from build123d import *

# Parameters (mm, degrees)
SKETCH1_R           = 1.625
BOSS_EXTRUDE1_DEPTH = 6.35


with BuildPart() as part:
    # Sketch1 → Boss-Extrude1 (new body)
    with BuildSketch(Plane(origin=(0, 0, 0), x_dir=(1, 0, 0), z_dir=(0, 1, 0))):
        with BuildLine():
            ThreePointArc((50.8, 0), (13.148007491, 49.069031975), (-43.994090512, 25.4))
            ThreePointArc((-43.994090512, 25.4), (-43.585026823, 18.428634878), (-37.019722443, 16.048709846))
            ThreePointArc((-37.019722443, 16.048709846), (-35.546093598, 16.258298381), (-34.059144925, 16.191268754))
            ThreePointArc((-34.059144925, 16.191268754), (-31.463683221, 17.007149664), (-30.452841612, 19.533071743))
            ThreePointArc((-30.452841612, 19.533071743), (-30.028839685, 22.644562363), (-28.439901214, 25.353146135))
            ThreePointArc((-28.439901214, 25.353146135), (13.565577093, 35.603161631), (38.1, 0))
            ThreePointArc((38.1, 0), (44.45, -6.35), (50.8, 0))
        make_face()
        with Locations((-38.494829198, 22.225)):
            Circle(SKETCH1_R, mode=Mode.SUBTRACT)
        with Locations((44.45, 0)):
            Circle(SKETCH1_R, mode=Mode.SUBTRACT)
        with Locations((11.504506555, 42.935402979)):
            Circle(SKETCH1_R, mode=Mode.SUBTRACT)
    extrude(amount=BOSS_EXTRUDE1_DEPTH)


solid = part.part
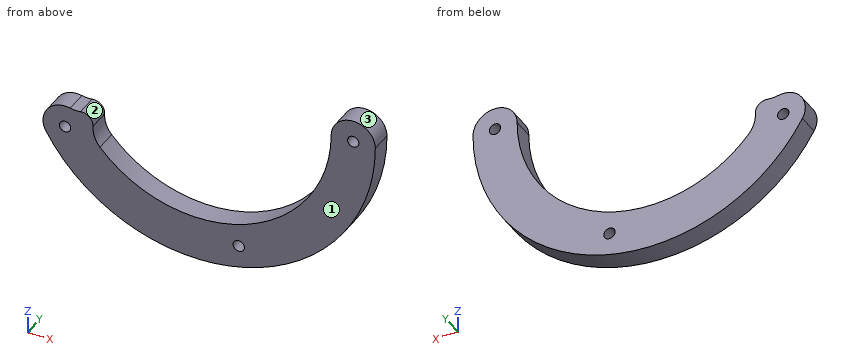
Could you check a few things on this model? Use its own coordinates, in mm. Face numbers are marked on the shaded views. Give positions to 0.01 mm unless a question says otherwise; leave off trailing zeros. Write each loop counter-clockwise with the first axis right and the second up, starting at its lowest first coordinate (ties: lowest second). Pieces come first, ordered by that corner, then holes. Notation, with made-up numbers: (88.25, -36.5) -> (93.25, -36.5) arc R28 ccw to (93.25, 1.5) -> close; hole circle Ø10 at (17.25, 48.5). An arc over 180 degrees is marked (long way). Answer as CSV lines item,"result". Start each with the question number.
(1) If we section it at B-B, the plane x = 44.45: Write out the boundary of the cut face in (y, z) (3 decimals), and give its area (3 significant figures).
(2) I'm going to push flat-ended pins straight in: pin 1 Ø1.5 at (y, z) = (4.5, -20) entering from +X; pin 2 Ø3 at (x, z) = (44.45, 0) entering from +Y; pin 3 Ø12 at (x, z) = (-28.5, -21.5) entering from +Y; pin 4 Ø2 at (y, z) = (3, -13) entering from +X. Where does each tip first touch, or does it pass through?
(3) If we section it at D-D, the plane z = -5.5: Write out the boundary of the cut face in (x, y), and give its area (3 significant figures).
(4) If we section it at A-A, the plane z = -31: Write out the boundary of the cut face in (x, y), and give its area (3 significant figures).
(5) If we section it at C-C, the plane y = 1: Give the number of separate pieces and of enclosed holes in the cut face, and give its area (3 significant figures).
(6) Please list where these lines run through material, in increasing order: line 1 (Z direction, x = 44.45, y = 1.5) (3 decimals); line 2 (Z direction, x = 44.5, y = 2); line 3 (X direction, y = 5.75, z = -26.5).
(7) If we mould it in two halves opening along X, with no side actions, what happens to the marked faces 1, 2 and 3? For each: +X half, -X half, draft (parallel to the pull), parting line (faces both ways), or undercut.
Answer list:
1,outline,"(0, -24.593) -> (6.35, -24.593) -> (6.35, -1.625) -> (0, -1.625) -> close; (0, 1.625) -> (6.35, 1.625) -> (6.35, 6.35) -> (0, 6.35) -> close"
1,area,"176 mm^2"
2,pin 1,"x = 47.01"
2,pin 2,"through"
2,pin 3,"y = 6.35"
2,pin 4,"x = 49.36"
3,outline,"(37.7, 0) -> (50.5, 0) -> (50.5, 6.35) -> (37.7, 6.35) -> close"
3,area,"81.3 mm^2"
4,outline,"(-40.24, 0) -> (-22.15, 0) -> (-22.15, 6.35) -> (-40.24, 6.35) -> close; (22.15, 0) -> (40.24, 0) -> (40.24, 6.35) -> (22.15, 6.35) -> close"
4,area,"230 mm^2"
5,separate pieces,"1"
5,enclosed holes,"3"
5,area,"1,590 mm^2"
6,line 1,"-24.593 to -1.625, 1.625 to 6.35"
6,line 2,"-24.5 to -1.62, 1.62 to 6.35"
6,line 3,"-43.34 to -27.37, 27.37 to 43.34"
7,face 1,"draft"
7,face 2,"undercut"
7,face 3,"parting line"
